Work out the finished part from the listing and answer in its coordinate system (mm). Coordinates: 2 decimals unless noted, no trailing zeros. Loops run counter-clockwise (first coordinate to the right, second up) from the corner with the lowest first, then second, coordinate; pieces in that order, holes last.
```python
from build123d import *

# Parameters (mm, degrees)
F0_W     = 150
F0_H     = 100
F0_R     = 10
F1_DEPTH = 20
F2_R     = 5
F3_SIZE  = 2
F5_D     = 4.2


with BuildPart() as f1:
    # F0 (on Top) → F1 (new body)
    with BuildSketch(Plane.XY):
        Rectangle(F0_W, F0_H)
        Circle(F0_R, mode=Mode.SUBTRACT)
    extrude(amount=F1_DEPTH)

    # F2
    f2_edges = [f1.edges().sort_by_distance(p)[0] for p in [
        (-75, -50, 10),
        (-75, 50, 10),
        (75, -50, 10),
        (75, 50, 10),
    ]]
    fillet(f2_edges, radius=F2_R)

    # F3
    f3_edges = [f1.edges().sort_by_distance(p)[0] for p in [
        (-10, 0, 0),
        (-10, 0, 20),
    ]]
    chamfer(f3_edges, length=F3_SIZE)

    # F5 (through all)
    with Locations(Plane(origin=(0, 0, 0), x_dir=(1, 0, 0), z_dir=(0, 0, -1))):
        with Locations((60, -37.5), (-60, -37.5), (-60, 37.5), (60, 37.5)):
            Hole(F5_D / 2)


solid = f1.part
```
1. A cutting plane is placed at A-A, the plane x = 60. Give the vertices of the cut face in (y, z), then the cut area to 3 significant figures.
2. A cutting plane is placed at D-D, the plane y = 0. Give the vertices of the cut face in (x, z), then the cut area to 3 significant figures.
3. This flat-tipped pin is pushed along its axis until it touches: P1, Ø23, axis at x = 0, y = 0, coming from the +Z side. Where does it stop, or does it pass through?
4. Straight lines are drawn through the part: probe 1 along X at (y, z) = (37.5, 6); probe 2 along Y at (x, z) = (-60, 4); probe 3 along Y at (x, z) = (0, 11.5). For each, find the intervals that lie inside material, in ascending order.
5. A cutting plane is placed at C-C, the plane x = 0. Give the vertices of the cut face in (y, z).
6. A cutting plane is placed at B-B, the plane y = -37.5. Give the vertices of the cut face in (x, z).
7. Determine the mould class of faces 1 (the cylindrical face through (-60.969, 39.363, 10.14)), 2 (the cylindrical face through (-74, 48, 10)), 3 (the flat face through (-1, -50, 10)) for opening direction X: released by +X, released by -X, zero draft, split by the parting line, or undercut.
Answers below:
1. outline: (-50, 0) - (-39.6, 0) - (-39.6, 20) - (-50, 20) - close; (-35.4, 0) - (35.4, 0) - (35.4, 20) - (-35.4, 20) - close; (39.6, 0) - (50, 0) - (50, 20) - (39.6, 20) - close
1. area: 1,830 mm2
2. outline: (-75, 0) - (-12, 0) - (-10, 2) - (-10, 18) - (-12, 20) - (-75, 20) - close; (10, 2) - (12, 0) - (75, 0) - (75, 20) - (12, 20) - (10, 18) - close
2. area: 2,590 mm2
3. P1: stops at z = 19.5
4. probe 1: x = -75 to -62.1, -57.9 to 57.9, 62.1 to 75
4. probe 2: y = -50 to -39.6, -35.4 to 35.4, 39.6 to 50
4. probe 3: y = -50 to -10, 10 to 50
5. outline: (-50, 0) - (-12, 0) - (-10, 2) - (-10, 18) - (-12, 20) - (-50, 20) - close; (10, 2) - (12, 0) - (50, 0) - (50, 20) - (12, 20) - (10, 18) - close
6. outline: (-75, 0) - (-62.1, 0) - (-62.1, 20) - (-75, 20) - close; (-57.9, 0) - (57.9, 0) - (57.9, 20) - (-57.9, 20) - close; (62.1, 0) - (75, 0) - (75, 20) - (62.1, 20) - close
7. face 1: undercut
7. face 2: released by -X
7. face 3: zero draft
